```python
from build123d import *

# Parameters (mm, degrees)
BOSS_EXTRUDE1_DEPTH = 290
SKETCH3_W           = 137
SKETCH3_H           = 57.4
SKETCH3_W_2         = 56
SKETCH3_H_2         = 30.6
BOSS_EXTRUDE2_DEPTH = 12.30416804
SKETCH3_3_W         = 121.3
SKETCH3_3_H         = 161.2
CUT_EXTRUDE1_DEPTH  = 307.006700561
CUT_EXTRUDE1_TAPER  = -35
SKETCH3_5_R         = 2
CUT_EXTRUDE2_DEPTH  = 307.006700694
CUT_EXTRUDE2_DRAFT  = 36
FILLET2_R           = 1


with BuildPart() as part:
    # Sketch1 → Boss-Extrude1 (new body)
    with BuildSketch(Plane(origin=(0, 0, 0), x_dir=(1, 0, 0), z_dir=(0, 1, 0))):
        with BuildLine():
            Line((0, 0), (-68.5, 0))
            Line((-68.5, 0), (-68.5, 7.5))
            Line((-68.5, 7.5), (-68.5, 12.30416804))
            Line((-68.5, 12.30416804), (-95, 12.30416804))
            ThreePointArc((-95, 12.30416804), (0, -22.69583196), (95, 12.30416804))
            Line((95, 12.30416804), (68.5, 12.30416804))
            Line((68.5, 12.30416804), (68.5, 7.5))
            Line((68.5, 7.5), (68.5, 0))
            Line((68.5, 0), (0, 0))
        make_face()
    extrude(amount=BOSS_EXTRUDE1_DEPTH)

    # Sketch3 → Boss-Extrude2 (add)
    with BuildSketch(Plane(origin=(0, 0, 0), x_dir=(-1, 0, 0), z_dir=(0, 0, -1))):
        with Locations((0, 261.3)):
            Rectangle(SKETCH3_W, SKETCH3_H)
        with Locations((-40.5, 15.3)):
            Rectangle(SKETCH3_W_2, SKETCH3_H_2)
        with Locations((40.5, 15.3)):
            Rectangle(SKETCH3_W_2, SKETCH3_H_2)
    extrude(amount=BOSS_EXTRUDE2_DEPTH)

    # Sketch3<3> → Cut-Extrude1 (cut, through all)
    with BuildSketch(Plane(origin=(0, 0, 0), x_dir=(-1, 0, 0), z_dir=(0, 0, -1))):
        with Locations((0, 130.6)):
            Rectangle(SKETCH3_3_W, SKETCH3_3_H)
    extrude(amount=-CUT_EXTRUDE1_DEPTH, taper=CUT_EXTRUDE1_TAPER, mode=Mode.SUBTRACT)


with BuildPart() as cut_extrude2_tool:
    # Sketch3<5> → Cut-Extrude2 (with draft: the straight prism first)
    with BuildSketch(Plane(origin=(0, 0, 0), x_dir=(-1, 0, 0), z_dir=(0, 0, -1))):
        with Locations((0, 220)):
            Circle(SKETCH3_5_R)
    extrude(amount=-CUT_EXTRUDE2_DEPTH)
    # Cut-Extrude2: the draft: its side faces are tilted about the plane it starts from
    cut_extrude2_sides = [cut_extrude2_tool.faces().sort_by_distance(p)[0] for p in [
        (2, 220, 153.503350347),
    ]]
    draft(cut_extrude2_sides, Plane(origin=(0, 0, 0), x_dir=(-1, 0, 0), z_dir=(0, 0, -1)), CUT_EXTRUDE2_DRAFT)


with BuildPart() as part_1:
    add(part.part)

    # Cut-Extrude2: cut by cut_extrude2_tool
    add(cut_extrude2_tool.part, mode=Mode.SUBTRACT)

    # Fillet2
    fillet2_edges = [part_1.edges().sort_by_distance(p)[0] for p in [
        (2, 220, 0),
    ]]
    fillet(fillet2_edges, radius=FILLET2_R)


solid = part_1.part
```
Can you work these out from the model? Positions are in its coordinate system, mm. A direction names the side the tool comes from. Give positions to 0.01 mm unless a question says otherwise; leave off trailing zeros. Loops run counter-clockwise (first coordinate to the right, second up) from the corner with the lowest first, then second, coordinate; pieces in that order, holes last. Notation, with made-up numbers: M -28,-37.75 L 4,-37.75 A17 ccw 4,-27.75 Z; hole C 41.25,48 d11. An arc over 180 degrees is marked long. Use one line per item in the form item = value. Start each with the question number.
(1) Please list where these lines run through material, in increasing order: line 1 (Y direction, x = 56, z = -9); line 2 (X direction, y = 44.5, z = -7); line 3 (X direction, y = 178.5, z = 7).
(2) I want a section at B-B, the plane x = 0. State how many separate pieces and enclosed holes the cut face has, and give its area (3 significant figures).
(3) I want a section at C-C, the plane y = 242. Write out the boundary of the cut face in (x, z), and give its area (3 significant figures).
(4) I'm going to push flat-ended pins straight in: P1, Ø10, axis at y = 127.5, z = 7.5, coming from the -X side; P2, Ø3.5, axis at y = 17, z = -3, coming from the +X side; P3, Ø3.5, axis at y = 137.5, z = -7, coming from the -X side. Where does each tip first touch, or does it pass through?
(5) Thinking about a two-plate mould opening in Y: for faces 4 (the flat face through (12.5, 15, -6)), 5 (the flat face through (-1, 0, 1)), 6 (the flat face through (-68.5, 130, -6)), which applies, released by +Y, released by -Y, zero draft, split by the parting line, or undercut?
(6) On a 3-axis mill with a long thin cutter (end or side, diameter ignored), from which of +Z, -Z, +X, -X, +Y, -Y can I reach the whole of each face in a straight line? I mean faces 1 (the flat face through (-12.5, 15, -6)), 2 (the flat face through (1, 244, -12.304)), 3 (the flat face through (68.5, 130, -6)). Say none if no direction works.
(7) I want a section at A-A, the plane z = -4. Write out the boundary of the cut face in (x, y), and give its area (3 significant figures).
Worked out:
q1.line_1 = 0 to 30.6, 232.6 to 290
q1.line_2 = -88.4 to -68.5, 68.5 to 88.4
q1.line_3 = -65.96 to -65.55, 65.55 to 65.96
q2.separate_pieces = 3
q2.enclosed_holes = 0
q2.area = 3,030 mm²
q3.outline = M -95,-12.3 L 95,-12.3 A146.43 ccw Z
q3.area = 4,550 mm²
q4.P1 = -74.21
q4.P2 = 85.35
q4.P3 = -90.67
q5.face_4 = zero draft
q5.face_5 = released by -Y
q5.face_6 = undercut
q6.face_1 = -Z, -Y
q6.face_2 = -Z, +X, -X, +Y, -Y
q6.face_3 = -Z
q7.outline = M -84.29,0 L -12.5,0 L -12.5,30.6 L -68.5,30.6 L -68.5,232.6 L 68.5,232.6 L 68.5,30.6 L 12.5,30.6 L 12.5,0 L 84.29,0 L 84.29,290 L -84.29,290 Z
q7.area = 20,500 mm²
